Here's how the part is built. I have some questions about the finished solid (model axes, mm). A direction names the side the tool comes from. Coordinates: 2 decimals unless noted, no trailing zeros. Loops run counter-clockwise (first coordinate to the right, second up) from the corner with the lowest first, then second, coordinate; pieces in that order, holes last. Notation, with made-up numbers: (71.5, 5.5) -> (129.5, 5.5) arc R30 cw to (129.5, 35.5) -> close; hole circle Ø10 at (70, -40). An arc over 180 degrees is marked (long way). Answer as a JSON object with one key per item and string values. Group by question number.
1) Which directions (+Z, -Z, +X, -X, +Y, -Y) give clear straight access to the entire face, cutting with the end or side of a thin tool? Please do faces 5 (the cylindrical face through (-29.035, 39.412, -24.825)), 6 (the flat face through (1, 12, 37.5)), 7 (the flat face through (-5, 5, 1)), 8 (the cylindrical face through (12.24, 133.14, -0.18)).
2) I want a section at C-C (x = -3). Write out the boundary of the cut face in (y, z), then the cut area to 3 significant figures.
3) I want a section at A-A (z = -8.5). Write out the boundary of the cut face in (x, y), then the cut area to 3 significant figures.
4) I need wall thicknesses on probe 1 along Y at (x, z) = (4.5, -17.5); probe 2 along Y at (x, z) = (-3, 11.5); probe 3 along Z at (x, y) = (34.5, 26). Which ranges of each line are inside material? Lowest first, please. Write a range as [from, to].
5) I'm going to push flat-ended pins straight in: pin 1 (20 mm diameter, centred on x = -11.5, z = -24.5, fed in from +Y); pin 2 (1.5 mm diameter, centred on y = 152, z = -12.5, fed in from -X); pin 3 (6 mm diameter, centred on x = 18, y = 101.5, fed in from +Z); pin 4 (1.5 mm diameter, centred on x = -27, z = 3.5, fed in from -Y). Where does each tip first touch, or does it pass through?
6) I want a section at D-D (z = 29). Write out the boundary of the cut face in (x, y), then the cut area to 3 significant figures.
7) If we mould it in two halves opening along X, with no side actions, what happens to faces 1 (the flat face through (1, 25, 13)), 2 (the flat face through (-24.74, 64.16, -24.82)), 3 (the flat face through (39.74, 90.93, -24.82)), 4 (the cylindrical face through (6.46, 137.99, -12.85))? For each: +X half, -X half, draft (parallel to the pull), parting line (faces both ways), or undercut.
8) I want a section at B-B (y = 142). Write out the boundary of the cut face in (x, z).
Autodesk Inventor part; units mm, degrees
ref_plane "YZ Plane" through (0, 0, 0) normal (1, 0, 0) x (0, 1, 0)
ref_plane "XZ Plane" through (0, 0, 0) normal (0, 1, 0) x (-1, 0, 0)
ref_plane "XY Plane" through (0, 0, 0) normal (0, 0, 1) x (1, 0, 0)
sketch "Szkic1" plane through (0, 0, 0) normal (0, 1, 0) x (-1, 0, 0)
  line L0 (56, -37.5) -> (-56, -37.5)
  line L1 (-56, -37.5) -> (-56, 37.5)
  line L2 (-56, 37.5) -> (56, 37.5)
  line L3 (56, 37.5) -> (56, -37.5)
  line L4 (56, -37.5) -> (-56, 37.5) construction
  line L5 (-56, -37.5) -> (56, 37.5) construction
  point P0 (0, 0)
  dimension "d0" = 112
  dimension "d1" = 75
extrude "Wyciągnięcie proste1" add sketch "Szkic1" along normal blind 25
sketch "Szkic2" plane through (0, 25, 0) normal (0, 1, 0) x (1, 0, 0)
  line L0 (56, 37.5) -> (-56, 37.5)
  line L1 (56, -37.5) -> (56, 37.5)
  line L2 (-56, 37.5) -> (56, 37.5)
  line L3 (56, 37.5) -> (56, 12.5)
  line L4 (56, 12.5) -> (-56, 12.5)
  line L5 (-56, 12.5) -> (-56, 37.5)
  point P0 (0, 0)
  dimension "d4" = 25
extrude "Wyciągnięcie proste2" add sketch "Szkic2" along normal blind 148
sketch "Szkic3" plane through (-56, 25, -12.5) normal (0, 0, 1) x (1, 0, 0)
  circle A0 centre (57.4852, 125) radius 23
  line L0 (0, 0) -> (112, 0)
  line L1 (112, -25) -> (112, 148)
  line L2 (0, -25) -> (0, 148)
  line L3 (0, 0) -> (0, 148)
  line L4 (0, 148) -> (112, 148)
  line L5 (0, 148) -> (112, 148)
  line L6 (112, 148) -> (112, 0)
  line L7 (0, 0) -> (35.2766, 130.9813)
  line L8 (79.6938, 130.9813) -> (112, 0)
  point P0 (56, -25)
  point P1 (79.928, 130.0318)
  point P2 (57.4852, 148)
  dimension "d8" = 46
extrude "Wyciągnięcie proste3" cut sketch "Szkic3" against normal blind 25 contours L7 L2 L4 A0 | L4 L1 L8 A0
sketch "Szkic4" plane through (-56, 25, -12.5) normal (0, 0, 1) x (1, 0, 0)
  arc A0 (79.928, 130.0318) -> (35.2766, 130.9813) centre (57.4852, 125) ccw
  circle A1 centre (57.4852, 125) radius 20
  point P0 (56, -25)
  dimension "d11" = 40
extrude "Wyciągnięcie proste4" add sketch "Szkic4" along normal blind 25
sketch "Szkic5" plane through (-56, 25, -12.5) normal (0, 0, 1) x (1, 0, 0)
  line L0 (56, 12) -> (31.7743, 12)
  line L1 (25.9808, 19.5604) -> (42.2104, 79.8208)
  line L2 (0, 0) -> (112, 0)
  line L3 (35.2766, 130.9813) -> (0, 0)
  arc A0 (25.9808, 19.5604) -> (31.7743, 12) centre (31.7743, 18) ccw
  circle A1 centre (57.4852, 125) radius 20
  line L4 (56, 12) -> (80.2257, 12)
  line L5 (86.0192, 19.5604) -> (69.7896, 79.8208)
  arc A2 (80.2257, 12) -> (86.0192, 19.5604) centre (80.2257, 18) ccw
  circle A3 centre (56, 54.1155) radius 20
  point P0 (56, -25)
  point P1 (75.3119, 59.3167)
  point P2 (36.6881, 59.3167)
  dimension "d14" = 12
  dimension "d15" = 20
  dimension "d16" = 6
  dimension "d17" = 40
extrude "Wyciągnięcie proste5" cut sketch "Szkic5" against normal blind 25 contours L0 A0 L1 A3 L5 A2 L4 | A3
sketch "Szkic6" plane through (1.4852, 150, 12.5) normal (0, 0, 1) x (1, 0, 0)
  point P0 (-1.4852, -150)
  point P1 (0, 0)
hole "Otwór1" at (1.4852, 150, 12.5) direction (0, 0, -1) diameter 26 end through all
sketch "Szkic7" plane through (0, 0, 0) normal (0, -1, 0) x (1, 0, 0)
  point P0 (0, 0)
sketch "Szkic8" plane through (-56, 0, 37.5) normal (0, 0, 1) x (1, 0, 0)
  line L0 (112, 0) -> (0, 0)
  line L1 (46, 0) -> (66, 0)
  line L2 (0, 0) -> (112, 0)
  line L3 (46, 0) -> (56, 10)
  line L4 (46, 0) -> (60.1421, 0) construction
  line L5 (56, 10) -> (66, 0)
  point P0 (56, 0)
  dimension "d27" = 20
  dimension "d28" = 45
extrude "Wyciągnięcie proste6" cut sketch "Szkic8" against normal blind 75
Determined:
{
 "1": {"face 5": "+Z, -Z", "face 6": "+Z, +X, -X, +Y, -Y", "face 7": "+Z, -Z, -Y", "face 8": "+Z"},
 "2": {"outline": "(7, -37.5) -> (37, -37.5) -> (37, -12.5) -> (25, -12.5) -> (25, 37.5) -> (7, 37.5) -> close; (98.89, -37.5) -> (137.8, -37.5) -> (137.8, 12.5) -> (130.51, 12.5) -> (130.51, -12.5) -> (98.89, -12.5) -> close; (162.2, -37.5) -> (172.56, -37.5) -> (172.56, -12.5) -> (169.49, -12.5) -> (169.49, 12.5) -> (162.2, 12.5) -> close", "area": "3,250 mm^2"},
 "3": {"outline": "(-56, 0) -> (-10, 0) -> (0, 10) -> (10, 0) -> (56, 0) -> (56, 25) -> (-56, 25) -> close; circle Ø40 at (1.49, 150); hole circle Ø26 at (1.49, 150)", "area": "3,430 mm^2"},
 "4": {"probe 1": "[5.5, 37], [98.6, 137.35], [162.65, 172.8]", "probe 2": "[7, 25], [130.51, 137.8], [162.2, 169.49]", "probe 3": "[-37.5, -12.5]"},
 "5": {"pin 1": "y = 172.81", "pin 2": "x = -22", "pin 3": "z = -12.5", "pin 4": "y = 0"},
 "6": {"outline": "(-56, 0) -> (-10, 0) -> (0, 10) -> (10, 0) -> (56, 0) -> (56, 25) -> (-56, 25) -> close", "area": "2,700 mm^2"},
 "7": {"face 1": "draft", "face 2": "undercut", "face 3": "+X half", "face 4": "undercut"},
 "8": {"outline": "(-24.49, -37.5) -> (-8.76, -37.5) -> (-8.76, 12.5) -> (-16.85, 12.5) -> (-16.85, -12.5) -> (-24.49, -12.5) -> close; (11.73, -37.5) -> (27.14, -37.5) -> (27.14, -12.5) -> (19.82, -12.5) -> (19.82, 12.5) -> (11.73, 12.5) -> close"}
}
